Geometry check sheet. Reference: the model listing, model coordinates, mm. A direction names the side the tool comes from. Round coordinates to 2 decimals unless told otherwise and drop trailing zeros. Use a Markdown table: item, result. Add a question column.
Item 1: Material ranges on probe 1 along X at (y, z) = (0, 1.5); probe 2 along Y at (x, z) = (7.5, -1.5); probe 3 along Y at (x, z) = (86.5, -3), recorded low to high. Write a range as [from, to].
Item 2: Set-up check for faces 4 (the flat face through (83, 37, 3.112)), 5 (the cylindrical face through (-31.41, 0.39, 2.36)), 6 (the flat face through (75, 33, -3.112)), 7 (the cylindrical face through (-32.757, 0.411, 0.022)): record each of +Z, -Z, +X, -X, +Y, -Y from which the full face is reachable in a straight line by a thin tool's end or side.
Item 3: Gauge pin test, flat ends, axial feed: pin 1 Ø1.5 at (y, z) = (4, 0.5) entering from +X; pin 2 Ø5 at (y, z) = (-7, -2) entering from +X; pin 3 Ø1 at (x, z) = (108.5, -1) entering from -Y. Record the tip position at first contact, or that the pin passes through.
Item 4: Mould release check, pull along Y, two halves, no side actions. Record for faces 1 (the cylindrical face through (201.03, 1.18, 0.02)), 2 (the flat face through (84, -35, -3.112)), 3 (the cylindrical face through (-37.39, -1.18, -2.36)): pulls with the +Y half, pulls with the -Y half, needs draft (parallel to the pull), parting line crosses it, or undercut.
Autodesk Inventor part; units mm, degrees
ref_plane "Work Plane2" through (0, 0, 0) normal (-1, 0, 0) x (0, 0, 1)
ref_plane "Work Plane3" through (168.275, 1.5875, 0) normal (-0.9957572, 0.0920191, 0) x (0, 0, 1)
ref_plane "Section Plane" through (0.3246, -34.409, 0) normal (0.9999555, 0.0094335, 0) x (0, 0, 1)
ref_plane "Work Plane2" through (0, 0, 0) normal (-1, 0, 0) x (0, 0, 1)
ref_plane "Work Plane3" through (168.275, 1.5875, 0) normal (-0.9957572, 0.0920191, 0) x (0, 0, 1)
sketch "Path" plane through (0, 0, 0) normal (0, 0, 1) x (1, 0, 0)
  arc A0 (-0.3246, 34.409) -> (0.3246, -34.409) centre (0, 0) ccw
  arc A1 (168.5996, -32.8215) -> (167.9504, 35.9965) centre (168.275, 1.5875) ccw
  line L0 (168.5996, -32.8215) -> (0.3246, -34.409)
  line L1 (-0.3246, 34.409) -> (167.9504, 35.9965)
  dimension "d31" = 5.9944
ref_plane "Section Plane" through (0.3246, -34.409, 0) normal (0.9999555, 0.0094335, 0) x (0, 0, 1)
sketch "Section Sketch" plane through (0.3246, -34.409, 0) normal (0.9999555, 0.0094335, 0) x (0, 0, 1)
  line L0 (-4.318, -1.1494) -> (4.318, -1.1494)
  line L1 (4.318, -1.1494) -> (4.318, 1.1494)
  line L2 (4.318, 1.1494) -> (-4.318, 1.1494)
  line L3 (-4.318, 1.1494) -> (-4.318, -1.1494)
  line L4 (-1.5875, -1.651) -> (1.5875, -1.651)
  line L5 (1.5875, -1.651) -> (1.5875, 1.651)
  line L6 (1.5875, 1.651) -> (-1.5875, 1.651)
  line L7 (-1.5875, 1.651) -> (-1.5875, -1.651)
  line L8 (-1.5875, 0) -> (1.5875, 0) construction
  line L9 (-3.1115, -2.9972) -> (-1.5875, -2.9972)
  line L10 (-1.5875, -2.9972) -> (-1.5875, 2.9972)
  line L11 (-1.5875, 2.9972) -> (-3.1115, 2.9972)
  line L12 (-3.1115, 2.9972) -> (-3.1115, -2.9972)
  line L13 (1.5875, -2.9972) -> (3.1115, -2.9972)
  line L14 (3.1115, -2.9972) -> (3.1115, 2.9972)
  line L15 (3.1115, 2.9972) -> (1.5875, 2.9972)
  line L16 (1.5875, 2.9972) -> (1.5875, -2.9972)
  line L17 (-4.318, 0) -> (4.318, 0) construction
  point P0 (0, 0)
  point P1 (0, 0)
  dimension "d21" = 2.2987
  dimension "d22" = 3.302
  dimension "d23" = 3.175
  dimension "d24" = 1.524
  dimension "d31" = 5.9944
  dimension "d32" = 8.636
sweep "Solid" add profiles "Section Sketch" path "Path"
pattern_of_one "Strand Pattern"
equation "\"d21\" = da_d2"
equation "\"d22\" = da_d1"
equation "\"d23\" = da_b1"
equation "\"d24\" = da_t1 + da_t2"
equation "\"d30\" = da_pt"
equation "\"da_p\" = 6.35"
equation "\"da_b1\" = 3.175"
equation "\"da_h2\" = 5.9944"
equation "\"da_h3\" = 5.207"
equation "\"da_d1\" = 3.302"
equation "\"da_d2\" = 2.2987"
equation "\"da_pt\" = 6.4008"
equation "\"da_b\" = 8.636"
equation "\"da_t1\" = 0.762"
equation "\"da_t2\" = 0.762"
properties part number "Roller Chain" material "Stainless Steel, 440C"
Found:
| question | item | result |
|---|---|---|
| 1 | probe 1 | x = [-36.06, -32.76], [201, 204.3] |
| 1 | probe 2 | y = [-35.99, -32.69], [32.83, 36.13] |
| 1 | probe 3 | y = [-36.59, -30.6], [32.23, 38.23] |
| 2 | face 4 | +Z |
| 2 | face 5 | +Z, -Z |
| 2 | face 6 | -Z |
| 2 | face 7 | none |
| 3 | pin 1 | stops at x = 204.3 |
| 3 | pin 2 | stops at x = 205.18 |
| 3 | pin 3 | stops at y = -35.04 |
| 4 | face 1 | undercut |
| 4 | face 2 | needs draft |
| 4 | face 3 | parting line crosses it |
